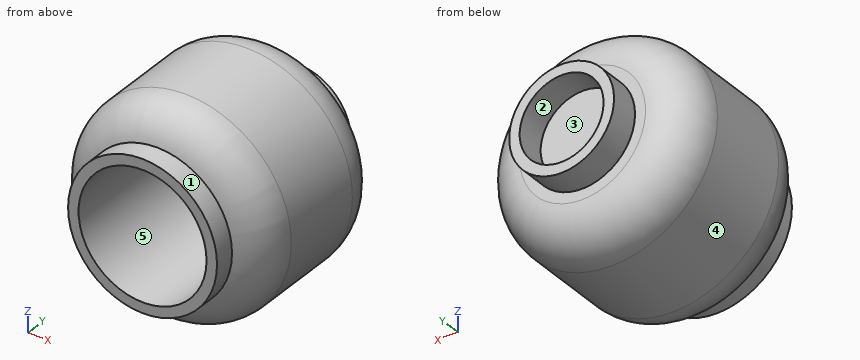
from build123d import *

# Parameters (mm, degrees)
F0_R     = 3.55
F0_R_2   = 3.05
F1_DEPTH = 1
F2_R     = 5
F3_DEPTH = 8
F5_R     = 2.5
F5_R_2   = 2
F6_DEPTH = 1.4
F8_DEPTH = 5


# Not quite as in the source:
# - a fillet or chamfer that OpenCascade refuses, or shapes differently, is made with other operations: its cross-section is extruded or revolved along the edge and cut away or added


with BuildPart() as f1:
    # F0 (on Front) → F1 (new body)
    with BuildSketch(Plane.XZ):
        Circle(F0_R)
        Circle(F0_R_2, mode=Mode.SUBTRACT)
    extrude(amount=F1_DEPTH)

    # F2 (on Front) → F3 (join)
    with BuildSketch(Plane.XZ):
        Circle(F2_R)
    extrude(amount=-F3_DEPTH)

    # F5 (on face) → F6 (join)
    with BuildSketch(Plane(origin=(0, 8, 0), x_dir=(-1, 0, 0), z_dir=(0, 1, 0))):
        Circle(F5_R)
        Circle(F5_R_2, mode=Mode.SUBTRACT)
    extrude(amount=F6_DEPTH)

    # F7: fillet of radius 2 on 2 edges, made by hand

    # F7_s1 → F7_t2 (revolve, cut)
    with BuildSketch(Plane.XY):
        with BuildLine():
            ThreePointArc((5, 6), (4.4142135624, 7.4142135624), (3, 8))
            Line((3, 8), (5, 8))
            Line((5, 8), (5, 6))
        make_face()
    revolve(axis=Axis((0, 8, 0), (0, -1, 0)), mode=Mode.SUBTRACT)

    # F7_s3 → F7_t4 (revolve, cut)
    with BuildSketch(Plane.XY):
        with BuildLine():
            ThreePointArc((5, 1.9228884523), (4.5968719423, 0.7187289944), (3.55, 0))
            Line((3.55, 0), (5, 0))
            Line((5, 0), (5, 1.9228884523))
        make_face()
    revolve(axis=Axis((0, 0, 0), (0, -1, 0)), mode=Mode.SUBTRACT)

    # F8 (cut): a face of the model
    f8_faces = [f1.faces().sort_by_distance(p)[0] for p in [
        (0, 0, 0),
    ]]
    extrude(f8_faces, amount=-F8_DEPTH, mode=Mode.SUBTRACT)


solid = f1.part
For this review, take the finished solid that the model builds, in its own axes (mm). Face numbers are marked on the shaded views. A direction names the side the tool comes from. Round coordinates to 2 decimals unless told otherwise and drop trailing zeros. Order: outer loops, then holes, each group sorted by start corner. A loop starts at its lowest first (then second) coordinate and runs counter-clockwise, first axis right, second up. Notation, with made-up numbers: M -4,51 L 42,51 A18 cw 42,62 Z; hole C 12.5,-39 d10. An arc over 180 degrees is marked long. Use a Markdown table: item, result. Add a question column.
Item 1: Add section C-C, the plane y = 0.75. Give the boundary of the cut face in (x, z), then the cut area to 3 significant figures.
Item 2: Add section B-B, the plane x = 0. Give the boundary of the cut face in (y, z).
Item 3: Add section A-A, the plane z = 0. Give the boundary of the cut face in (x, y), then the cut area to 3 significant figures.
Item 4: To check wall thickness, follow line 1 along Z through (x, y) = (0, 3); line 2 along Z through (x, y) = (0, 8.65); line 3 along Y through (x, z) = (0, 1.5). State the ranges of each line that lie inside material, in increasing order.
Item 5: Tool access review of the marked faces 3, 4 and 5: name each direction out of +Z, -Z, +X, -X, +Y, -Y from which nothing blocks a thin tool from reaching the whole face with its end or side.
Item 6: Mouldability with a two-part tool opening along X and no side actions: class the marked faces 1 and 2 as released by +X, released by -X, zero draft, split by the parting line, or undercut.
Item 7: Insertion check: pin 1 (2 mm diameter, centred on y = 0.5, z = -0.5, fed in from -X); pin 2 (5.5 mm diameter, centred on x = 0, z = 0, fed in from -Y); pin 3 (5 mm diameter, centred on x = -0.5, z = 1, fed in from +Y); pin 4 (1.5 mm diameter, centred on x = 0, y = 7, fed in from -Z). Each pin has a flat end and moves straight along its axis. Give the tip position at first contact, or say it passes through.
Geometry results:
| question | item | result |
|---|---|---|
| 1 | outline | C 0,0 d9.24; hole C 0,0 d6.1 |
| 1 | area | 37.8 mm² |
| 2 | outline | M -1,-3.55 L 0,-3.55 A2 ccw 1.92,-5 L 6,-5 A2 ccw 8,-3 L 8,-2.5 L 9.4,-2.5 L 9.4,-2 L 8,-2 L 8,2 L 9.4,2 L 9.4,2.5 L 8,2.5 L 8,3 A2 ccw 6,5 L 1.92,5 A2 ccw 0,3.55 L -1,3.55 L -1,3.05 L 5,3.05 L 5,-3.05 L -1,-3.05 Z |
| 3 | outline | M -5,1.92 A2 ccw -3.55,0 L -3.55,-1 L -3.05,-1 L -3.05,5 L 3.05,5 L 3.05,-1 L 3.55,-1 L 3.55,0 A2 ccw 5,1.92 L 5,6 A2 ccw 3,8 L 2.5,8 L 2.5,9.4 L 2,9.4 L 2,8 L -2,8 L -2,9.4 L -2.5,9.4 L -2.5,8 L -3,8 A2 ccw -5,6 Z |
| 3 | area | 48.7 mm² |
| 4 | line 1 | z = -5 to -3.05, 3.05 to 5 |
| 4 | line 2 | z = -2.5 to -2, 2 to 2.5 |
| 4 | line 3 | y = 5 to 8 |
| 5 | face 3 | +Y |
| 5 | face 4 | +Y, -Y |
| 5 | face 5 | -Y |
| 6 | face 1 | split by the parting line |
| 6 | face 2 | undercut |
| 7 | pin 1 | stops at x = -4.94 |
| 7 | pin 2 | stops at y = 5 |
| 7 | pin 3 | stops at y = 9.4 |
| 7 | pin 4 | stops at z = -4.98 |
